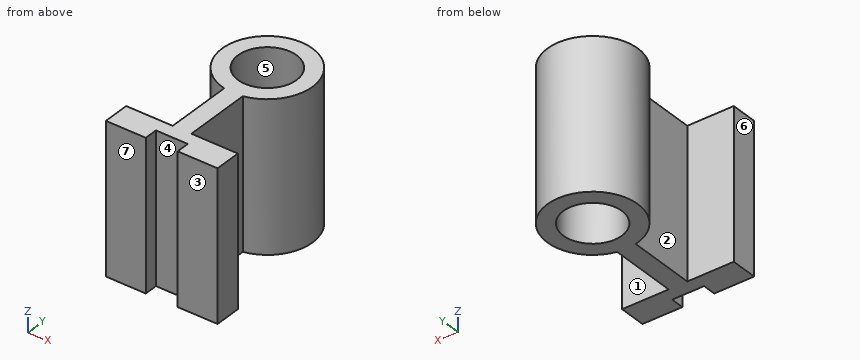
from build123d import *

# Parameters (mm, degrees)
F0_R     = 11
F1_DEPTH = 56


with BuildPart() as f1:
    # F0 (on Top) → F1 (new body)
    with BuildSketch(Plane.XY):
        with BuildLine():
            Line((0, 25.364195), (0, 0))
            Line((0, 0), (-17.5, 0))
            Line((-17.5, 0), (-17.5, -10))
            Line((-17.5, -10), (-2.5, -10))
            Line((-2.5, -10), (-2.5, -5))
            Line((-2.5, -5), (9.5, -5))
            Line((9.5, -5), (9.5, -10))
            Line((9.5, -10), (24.5, -10))
            Line((24.5, -10), (24.5, 0))
            Line((24.5, 0), (7, 0))
            Line((7, 0), (7, 25.364195))
            ThreePointArc((7, 25.364195), (3.5, 59), (0, 25.364195))
        make_face()
        with Locations((3.5, 42)):
            Circle(F0_R, mode=Mode.SUBTRACT)
    extrude(amount=F1_DEPTH)


solid = f1.part
The listing builds one solid part. Answer for the finished solid, in the listing's coordinates (mm). Face numbers are marked on the shaded views. A direction names the side the tool comes from. Give positions to 0.01 mm unless a question says otherwise; leave off trailing zeros. Write each loop counter-clockwise with the first axis right and the second up, starting at its lowest first coordinate (ties: lowest second). Pieces come first, ordered by that corner, then holes.
1) Find the intervals of material crossed by L1, parallel to X at y = 41.5, z = 17.5; L2, parallel to Y at x = 3, z = 37; L3, parallel to Y at x = -6, z = 13, in increasing order.
2) Section C-C (x = 3.5) is taken. Write down the section's boundary in (y, z), and give its area (3 significant figures).
3) Section B-B (z = 38) is taken. Write down the section's boundary in (x, y).
4) A tool of negligible diameter and unlimited length cuts with its end or side. For the marked faces 1, 2 and 3, from which of +Z, -Z, +X, -X, +Y, -Y can it reach the whole face along a straight path? Write none if from no direction.
5) For a pull along X with two mould halves and no side action, classify the marked faces 4, 5, 6 and 7 as pulls with the +X half, pulls with the -X half, needs draft (parallel to the pull), parting line crosses it, or undercut.
6) Given P1, Ø4, axis at y = 51, z = 42, coming from the +X side; P2, Ø5, axis at x = 11, z = 7.5, coming from the +Y side; P3, Ø5, axis at x = 20, z = 17, coming from the +Y side, each flat-ended and moving along its own axis, determine where each tip first touches the part or whether it passes through.
7) Section A-A (y = 42) is taken. Write down the section's boundary in (x, z), and give its area (3 significant figures).
8) Section D-D (x = -6) is taken. Write down the section's boundary in (y, z).
Response:
1. L1: x = -13.49 to -7.49, 14.49 to 20.49
1. L2: y = -5 to 31.01, 52.99 to 58.99
1. L3: y = -10 to 0, 27.9 to 36.45, 47.55 to 56.1
2. outline: (-5, 0) - (31, 0) - (31, 56) - (-5, 56) - close; (53, 0) - (59, 0) - (59, 56) - (53, 56) - close
2. area: 2,350 mm2
3. outline: (-17.5, -10) - (-2.5, -10) - (-2.5, -5) - (9.5, -5) - (9.5, -10) - (24.5, -10) - (24.5, 0) - (7, 0) - (7, 25.36) arc R17 ccw (long way) to (0, 25.36) - (0, 0) - (-17.5, 0) - close; hole circle Ø22 at (3.5, 42)
4. face 1: +Z, -Z, +X
4. face 2: +Z, -Z, -X
4. face 3: +Z, -Z, +X, -X, -Y
5. face 4: undercut
5. face 5: undercut
5. face 6: pulls with the -X half
5. face 7: needs draft
6. P1: stops at x = 18.99
6. P2: stops at y = 58.25
6. P3: stops at y = 51.64
7. outline: (-13.5, 0) - (-7.5, 0) - (-7.5, 56) - (-13.5, 56) - close; (14.5, 0) - (20.5, 0) - (20.5, 56) - (14.5, 56) - close
7. area: 672 mm2
8. outline: (-10, 0) - (0, 0) - (0, 56) - (-10, 56) - close; (27.9, 0) - (36.45, 0) - (36.45, 56) - (27.9, 56) - close; (47.55, 0) - (56.1, 0) - (56.1, 56) - (47.55, 56) - close
